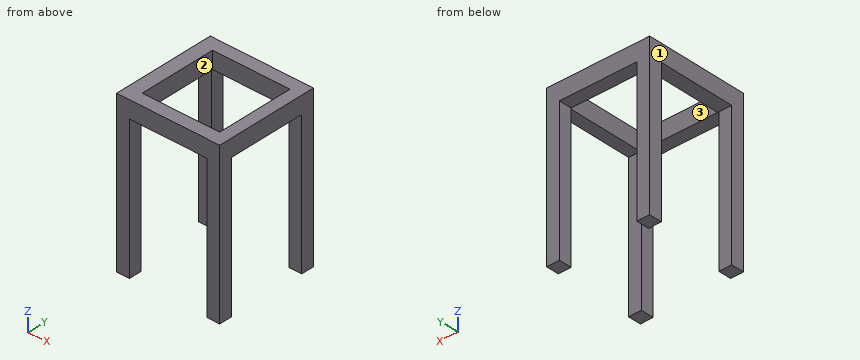
```python
from build123d import *

# Parameters (mm, degrees)
F0_W      = 120
F0_H      = 120
F1_DEPTH  = 5
F2_R      = 12.5
F3_DEPTH  = 25
F4_W      = 120
F4_H      = 120
F5_DEPTH  = 180
F6_W      = 90
F6_H      = 165
F7_DEPTH  = 120
F8_W      = 90
F8_H      = 165
F9_DEPTH  = 120
F10_W     = 90
F10_H     = 90
F11_DEPTH = 25


with BuildPart() as f1:
    # F0 (on Top) → F1 (new body)
    with BuildSketch(Plane.XY):
        with Locations((-0.624557, 27.300639)):
            Rectangle(F0_W, F0_H)
    extrude(amount=F1_DEPTH)

    # F2 (on face) → F3 (cut)
    with BuildSketch(Plane.XY.offset(5)):
        with Locations((-0.624557, 27.300639)):
            Circle(F2_R)
    extrude(amount=-F3_DEPTH, mode=Mode.SUBTRACT)

    # F4 (on face) → F5 (join)
    with BuildSketch(Plane.XY.offset(5)):
        with Locations((-0.624557, 27.300639)):
            Rectangle(F4_W, F4_H)
    extrude(amount=F5_DEPTH)

    # F6 (on face) → F7 (cut)
    with BuildSketch(Plane.XZ.offset(32.699361)):
        with Locations((-0.624557, 82.5)):
            Rectangle(F6_W, F6_H)
    extrude(amount=-F7_DEPTH, mode=Mode.SUBTRACT)

    # F8 (on face) → F9 (cut)
    with BuildSketch(Plane(origin=(-60.624557, 0, 0), x_dir=(0, -1, 0), z_dir=(-1, 0, 0))):
        with Locations((-27.300639, 82.5)):
            Rectangle(F8_W, F8_H)
    extrude(amount=-F9_DEPTH, mode=Mode.SUBTRACT)

    # F10 (on face) → F11 (cut)
    with BuildSketch(Plane.XY.offset(185)):
        with Locations((0.647055, 27.300639)):
            Rectangle(F10_W, F10_H)
    extrude(amount=-F11_DEPTH, mode=Mode.SUBTRACT)


solid = f1.part
```
Read the model definition and answer for the solid it produces. Units are mm, in the model's axes. Face numbers are marked on the shaded views. A direction names the side the tool comes from. Give positions to 0.01 mm unless a question says otherwise; leave off trailing zeros. Loops run counter-clockwise (first coordinate to the right, second up) from the corner with the lowest first, then second, coordinate; pieces in that order, holes last.
Item 1: The part is cut by section C-C (y = 39). Write down the section's boundary in (x, z), and give its area (3 significant figures).
Item 2: The part is cut by section B-B (x = 15). Write down the section's boundary in (y, z), and give its area (3 significant figures).
Item 3: For the marked faces 1, 2 and 3, determine the directions among +Z, -Z, +X, -X, +Y, -Y from which every point of the face is accessible in a straight line to the end or side of a thin tool.
Item 4: The part is cut by section D-D (x = -48.5). Write down the section's boundary in (y, z).
Item 5: The part is cut by section A-A (z = 41). Write down the section's boundary in (x, y).
Item 6: Find the intervals of material crossed by line 1 along Y through (x, z) = (-23, 173.5); line 2 along X through (y, z) = (31.5, 168); line 3 along X through (y, z) = (74, 62.5), in increasing order.
Item 7: Each of these flat-tipped pins is pushed along its axis until it touches: pin 1 Ø10 at (x, y) = (38.5, 4.5) entering from +Z; pin 2 Ø4 at (x, y) = (54, 49) entering from -Z. Where does it stop, or does it pass through?
Taken from the geometry:
1. outline: (-60.62, 165) - (-44.35, 165) - (-44.35, 185) - (-60.62, 185) - close; (45.65, 165) - (59.38, 165) - (59.38, 185) - (45.65, 185) - close
1. area: 600 mm2
2. outline: (-32.7, 165) - (-17.7, 165) - (-17.7, 185) - (-32.7, 185) - close; (72.3, 165) - (87.3, 165) - (87.3, 185) - (72.3, 185) - close
2. area: 600 mm2
3. face 1: +Z, -Z, -X, +Y, -Y
3. face 2: +Z, -Z
3. face 3: -Z
4. outline: (-32.7, 0) - (-17.7, 0) - (-17.7, 165) - (72.3, 165) - (72.3, 0) - (87.3, 0) - (87.3, 185) - (-32.7, 185) - close
5. outline: (-60.62, -32.7) - (-45.62, -32.7) - (-45.62, -17.7) - (-60.62, -17.7) - close; (-60.62, 72.3) - (-45.62, 72.3) - (-45.62, 87.3) - (-60.62, 87.3) - close; (44.38, -32.7) - (59.38, -32.7) - (59.38, -17.7) - (44.38, -17.7) - close; (44.38, 72.3) - (59.38, 72.3) - (59.38, 87.3) - (44.38, 87.3) - close
6. line 1: y = -32.7 to -17.7, 72.3 to 87.3
6. line 2: x = -60.62 to -44.35, 45.65 to 59.38
6. line 3: x = -60.62 to -45.62, 44.38 to 59.38
7. pin 1: passes through
7. pin 2: stops at z = 165
